Build history of the part. All positions in model axes, mm. A direction names the side the tool comes from. Give positions to 0.01 mm unless a question says otherwise; leave off trailing zeros. Order: outer loops, then holes, each group sorted by start corner. A loop starts at its lowest first (then second) coordinate and runs counter-clockwise, first axis right, second up. Notation, with made-up numbers: (-32.75, -4.5) - (-12.75, -4.5) arc R17 ccw to (-12.75, 12.5) - close; hole circle Ø2 at (48, 84.5). An arc over 180 degrees is marked (long way). Answer in a Markdown table with one row per item.
```python
from build123d import *

# Parameters (mm, degrees)
SKETCH_1_W          = 15
SKETCH_1_H          = 15
SKETCH_1_W_2        = 13
SKETCH_1_H_2        = 13
EXTRUDE_1_DEPTH     = 320
SKETCH_3_R          = 2
CUT_EXTRUDE_2_DEPTH = 321.43915179
SKETCH_4_R          = 2
CUT_EXTRUDE_3_DEPTH = 321.43915179
SKETCH_7_W          = 15
SKETCH_7_H          = 3
CUT_EXTRUDE_6_DEPTH = 20


with BuildPart() as part:
    # 草图1 → 凸台-拉伸1 (new body)
    with BuildSketch(Plane(origin=(0, 0, 0), x_dir=(1, 0, 0), z_dir=(0, 1, 0))):
        Rectangle(SKETCH_1_W, SKETCH_1_H)
        Rectangle(SKETCH_1_W_2, SKETCH_1_H_2, mode=Mode.SUBTRACT)
    extrude(amount=EXTRUDE_1_DEPTH)

    # 草图3 → 切除-拉伸2 (cut, through all)
    with BuildSketch(Plane.XY.offset(7.5)):
        with Locations((0, 295)):
            Circle(SKETCH_3_R)
        with Locations((0, 275)):
            Circle(SKETCH_3_R)
        with Locations(Location((0, 45, 0), (0, 0, 180))):
            Circle(SKETCH_3_R)
        with Locations(Location((0, 25, 0), (0, 0, 180))):
            Circle(SKETCH_3_R)
        with Locations((0, 255)):
            Circle(SKETCH_3_R)
        with Locations(Location((0, 65, 0), (0, 0, 180))):
            Circle(SKETCH_3_R)
    extrude(amount=-CUT_EXTRUDE_2_DEPTH, mode=Mode.SUBTRACT)

    # 草图4 → 切除-拉伸3 (cut, through all)
    with BuildSketch(Plane.ZY.offset(7.5)):
        with Locations((0, 8)):
            Circle(SKETCH_4_R)
        with Locations((0, 28)):
            Circle(SKETCH_4_R)
        with Locations(Location((0, 292, 0), (0, 0, 180))):
            Circle(SKETCH_4_R)
        with Locations(Location((0, 312, 0), (0, 0, 180))):
            Circle(SKETCH_4_R)
    extrude(amount=-CUT_EXTRUDE_3_DEPTH, mode=Mode.SUBTRACT)

    # 草图7 → 切除-拉伸6 (cut)
    with BuildSketch(Plane(origin=(7.5, 0, 0), x_dir=(0, 0, -1), z_dir=(1, 0, 0))):
        with Locations((0, 1.5)):
            Rectangle(SKETCH_7_W, SKETCH_7_H)
    extrude(amount=-CUT_EXTRUDE_6_DEPTH, mode=Mode.SUBTRACT)


solid = part.part
```
1. Which spindle directions (+Z, -Z, +X, -X, +Y, -Y) get a long thin tool onto all of the face, cutting with end or side? Do faces 1 (the face through (-6.5, 159, 0)), 2 (the face through (-7, 320, 0)). Say none if no direction does.
Check result:
| item | result |
|---|---|
| face 1 | +Y, -Y |
| face 2 | +Z, -Z, +X, -X, +Y |
2. Cut at A-A on y = 176. Write the cut outline in (x, z), and give its area (3 significant figures).
Check result:
| item | result |
|---|---|
| outline | (-7.5, -7.5) - (7.5, -7.5) - (7.5, 7.5) - (-7.5, 7.5) - close; hole (-6.5, -6.5) - (6.5, -6.5) - (6.5, 6.5) - (-6.5, 6.5) - close |
| area | 56.0 mm² |
3. Probe line 1 (Z direction, x = 3.25, y = 69); line 2 (Y direction, x = 7, z = 0). List the from-to ranges inside material, lowest first.
Check result:
| item | result |
|---|---|
| line 1 | z = -7.5 to -6.5, 6.5 to 7.5 |
| line 2 | y = 3 to 6, 10 to 26, 30 to 290, 294 to 310, 314 to 320 |
4. Drop a flat-ended pin along its axis: P1, Ø3.5, axis at y = 292, z = 0, coming from the +X side. Give the stop position or say it passes through.
Check result:
| item | result |
|---|---|
| P1 | passes through |
5. Two-plate mould, pull along Z, no slides. Class faces 3 (the face through (6.5, 159, 0)), 4 (the face through (0, 159, -7.5)), 5 (the face through (0, 159, 6.5)), 6 (the face through (0, 3, 7)): +Z half, -Z half, draft (parallel to the pull), parting line (faces both ways), or undercut.
Check result:
| item | result |
|---|---|
| face 3 | undercut |
| face 4 | -Z half |
| face 5 | undercut |
| face 6 | draft |
